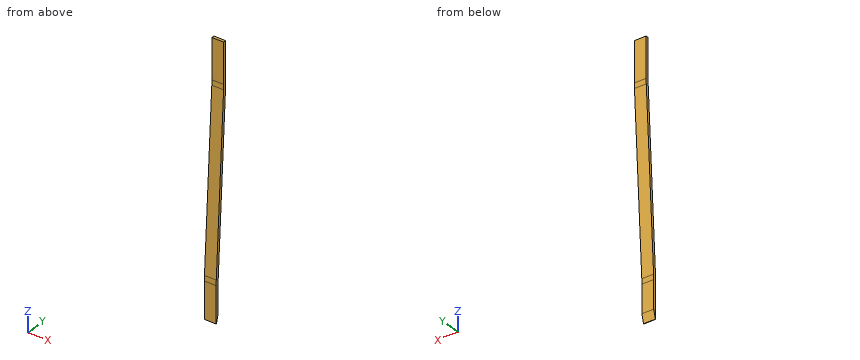
```python
from build123d import *

# Parameters (mm, degrees)
EXTRUDE1_DEPTH = 6.5


with BuildPart() as part:
    # Sketch1 → Extrude1 (new body, symmetric)
    with BuildSketch(Plane(origin=(0, 0, 0), x_dir=(0, 0, -1), z_dir=(1, 0, 0))):
        with BuildLine():
            Line((55, 14), (100, 14))
            ThreePointArc((100, 14), (102.839816619, 13.959669075), (105.67734259, 13.838708831))
            Line((105.67734259, 13.838708831), (302.152337132, 2.666129904))
            ThreePointArc((302.152337132, 2.666129904), (305.074988882, 2.541540853), (308, 2.5))
            Line((308, 2.5), (348.803847577, 2.5))
            Line((348.803847577, 2.5), (348.803847577, 3))
            Line((348.803847577, 3), (339.473720558, 5.5))
            Line((339.473720558, 5.5), (308, 5.5))
            ThreePointArc((308, 5.5), (305.160183381, 5.540330925), (302.32265741, 5.661291169))
            Line((302.32265741, 5.661291169), (105.847662868, 16.833870096))
            ThreePointArc((105.847662868, 16.833870096), (102.925011118, 16.958459147), (100, 17))
            Line((100, 17), (55, 17))
            Line((55, 17), (55, 14))
        make_face()
    extrude(amount=EXTRUDE1_DEPTH, both=True)


solid = part.part
```
For this review, take the finished solid that the model builds, in its own axes (mm). Coordinates: 2 decimals unless noted, no trailing zeros. Write each loop counter-clockwise with the first axis right and the second up, starting at its lowest first coordinate (ties: lowest second). Pieces come first, ordered by that corner, then holes.
(1) For pin 1 Ø6.5 at (x, z) = (-2, -323.5) entering from +Y; pin 2 Ø6.5 at (x, z) = (0, -79.5) entering from -Y; pin 3 Ø3 at (x, z) = (-1.5, -128.5) entering from -Y, all flat-tipped, find the tip position at first contact; note any pin that passes through.
(2) Wall thickness on probe 1 along Y at (x, z) = (-1.5, -311.5); probe 2 along Y at (x, z) = (0, -86): over which ranges is each line inside the solid? List them lowest first.
(3) Add section B-B on z = -76.5. Give the boundary of the cut face in (x, y), then the cut area to 3 significant figures.
(4) Add section C-C on y = 10. Give the boundary of the cut face in (x, z), then the cut area to 3 significant figures.
(5) Add section A-A on x = 4. Give the boundary of the cut face in (y, z), then the cut area to 3 significant figures.
Answer sheet:
1. pin 1: stops at y = 5.5
1. pin 2: stops at y = 14
1. pin 3: stops at y = 12.46
2. probe 1: y = 2.5 to 5.5
2. probe 2: y = 14 to 17
3. outline: (-6.5, 14) - (6.5, 14) - (6.5, 17) - (-6.5, 17) - close
3. area: 39.0 mm2
4. outline: (-6.5, -226.02) - (6.5, -226.02) - (6.5, -173.18) - (-6.5, -173.18) - close
4. area: 687 mm2
5. outline: (2.5, -348.8) - (3, -348.8) - (5.5, -339.47) - (5.5, -308) arc R100 cw to (5.66, -302.32) - (16.83, -105.85) arc R103 ccw to (17, -100) - (17, -55) - (14, -55) - (14, -100) arc R100 cw to (13.84, -105.68) - (2.67, -302.15) arc R103 ccw to (2.5, -308) - close
5. area: 871 mm2
